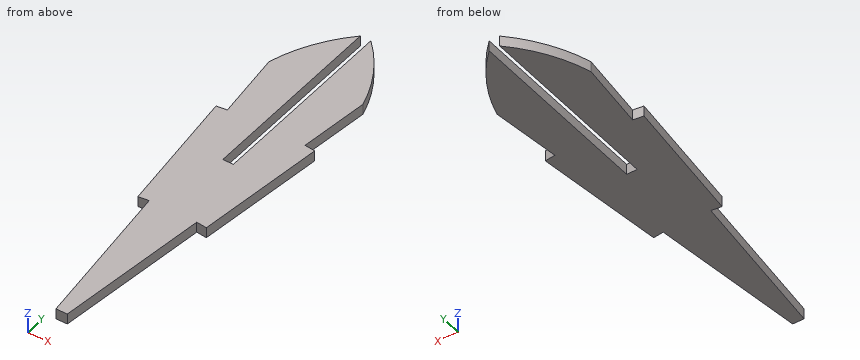
```python
from build123d import *

# Parameters (mm, degrees)
BOSS_EXTRUDE1_DEPTH = 1.524


with BuildPart() as part:
    # Sketch1 → Boss-Extrude1 (new body)
    with BuildSketch(Plane.XY):
        with BuildLine():
            Line((0, -185.062075144), (-1.524, -185.062075144))
            Line((-1.524, -185.062075144), (-1.524, -157.15233073))
            ThreePointArc((-1.524, -157.15233073), (-5.202982181, -161.792523258), (-7.537553978, -167.234588225))
            Line((-7.537553978, -167.234588225), (-6.374749179, -177.316845721))
            Line((-6.374749179, -177.316845721), (-7.888713502, -177.491453935))
            Line((-7.888713502, -177.491453935), (-5.70611082, -196.416007973))
            Line((-5.70611082, -196.416007973), (-4.192146497, -196.241399759))
            Line((-4.192146497, -196.241399759), (-1.585117021, -218.846004156))
            Line((-1.585117021, -218.846004156), (0.061117021, -218.846004156))
            Line((0.061117021, -218.846004156), (2.668146497, -196.241399759))
            Line((2.668146497, -196.241399759), (4.18211082, -196.416007973))
            Line((4.18211082, -196.416007973), (6.364713502, -177.491453935))
            Line((6.364713502, -177.491453935), (4.850749179, -177.316845721))
            Line((4.850749179, -177.316845721), (6.013553978, -167.234588225))
            ThreePointArc((6.013553978, -167.234588225), (3.678982181, -161.792523258), (0, -157.15233073))
            Line((0, -157.15233073), (0, -185.062075144))
        make_face()
    extrude(amount=BOSS_EXTRUDE1_DEPTH)


solid = part.part
```
Source: CAD feature listing. Evaluate the final solid. Frame: model axes, mm. Give positions to 0.01 mm unless a question says otherwise; leave off trailing zeros. Loops run counter-clockwise (first coordinate to the right, second up) from the corner with the lowest first, then second, coordinate; pieces in that order, holes last. Notation, with made-up numbers: (44, 41) -> (99, 41) arc R28 cw to (99, 75) -> close; hole circle Ø1 at (38.5, -5.5). An arc over 180 degrees is marked (long way). Use a Markdown table: item, result. Add a question column.
(1) Section query D-D (x = -0.75). Output: boundary loops of the cut face in (y, z), then the cut area to 3 significant figures.
(2) Section query A-A (z = 0.95). Output: boundary loops of the cut face in (x, y).
(3) Section query C-C (y = -168). Output: boundary loops of the cut face in (x, z).
(4) Ray query, line 1 (X direction, y = -162.5, z = 0.7); line 2 (X direction, y = -167.5, z = 0.65); line 3 (Y direction, x = -1, z = 0.2). Return the intervals inside material, ascending.
(5) Section query B-B (x = 5.5). Output: boundary loops of the cut face in (y, z), then the cut area to 3 significant figures.
Checked values:
| question | item | result |
|---|---|---|
| 1 | outline | (-218.85, 0) -> (-185.06, 0) -> (-185.06, 1.52) -> (-218.85, 1.52) -> close |
| 1 | area | 51.5 mm^2 |
| 2 | outline | (-7.89, -177.49) -> (-5.71, -196.42) -> (-4.19, -196.24) -> (-1.59, -218.85) -> (0.06, -218.85) -> (2.67, -196.24) -> (4.18, -196.42) -> (6.36, -177.49) -> (4.85, -177.32) -> (6.01, -167.23) arc R22.4 ccw to (0, -157.15) -> (0, -185.06) -> (-1.52, -185.06) -> (-1.52, -157.15) arc R22.4 ccw to (-7.54, -167.23) -> (-6.37, -177.32) -> close |
| 3 | outline | (-7.45, 0) -> (-1.52, 0) -> (-1.52, 1.52) -> (-7.45, 1.52) -> close; (0, 0) -> (5.93, 0) -> (5.93, 1.52) -> (0, 1.52) -> close |
| 4 | line 1 | -5.61 to -1.52, 0 to 4.08 |
| 4 | line 2 | -7.51 to -1.52, 0 to 5.98 |
| 4 | line 3 | -218.85 to -185.06 |
| 5 | outline | (-184.99, 0) -> (-177.39, 0) -> (-177.39, 1.52) -> (-184.99, 1.52) -> close; (-171.69, 0) -> (-165.63, 0) -> (-165.63, 1.52) -> (-171.69, 1.52) -> close |
| 5 | area | 20.8 mm^2 |
